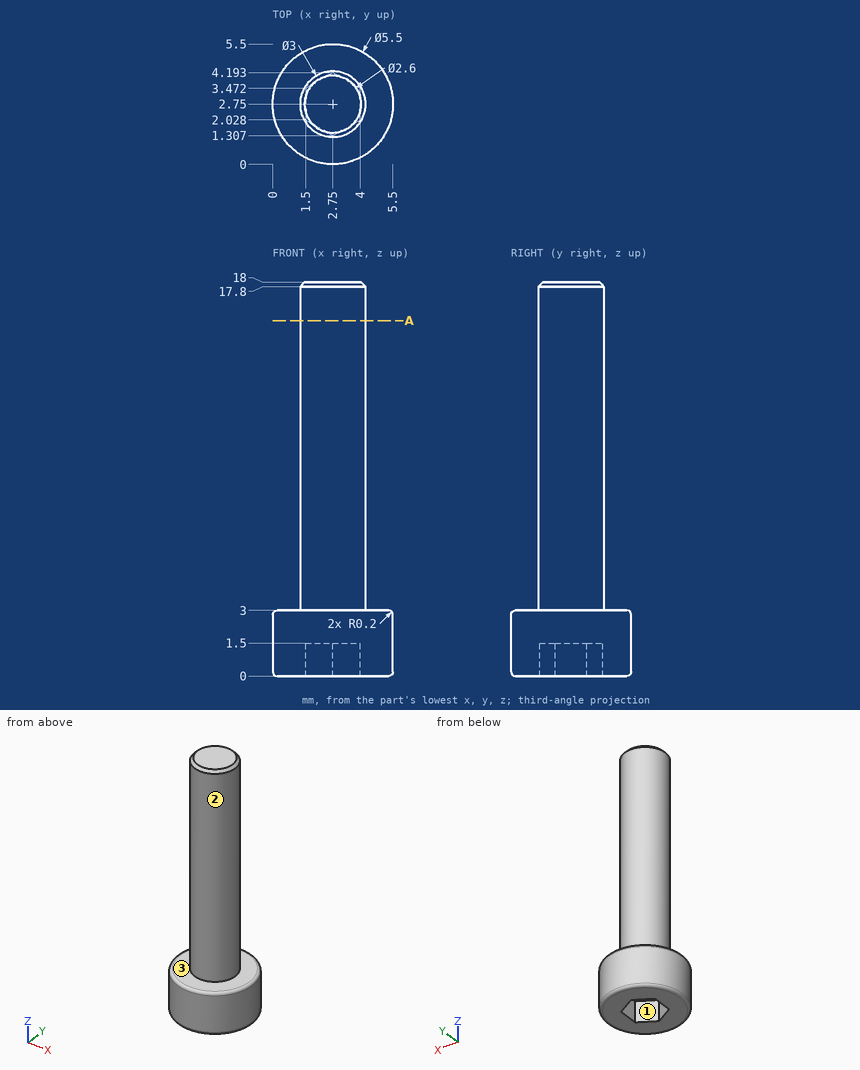
Here's the drawing with two shaded views (mm, measured from the low corner). I have some questions. Give positions to 0.01 mm unless a question says otherwise; leave off trailing zeros. Order: outer loops, then holes, each group sorted by start corner. A loop starts at its lowest first (then second) coordinate and runs counter-clockwise, first axis right, second up.
Q1. If I drill on line 1 along Z through (x, y) = (0.85, 4.4); line 2 along Z through (x, y) = (1.9, 2); line 3 along Y through (x, z) = (3.5, 2.5) (1 decimal), over which ranges is the centre line in solid material (lowest first)?
Q2. We'd pull the mould along X, two halves only. Please class the marked faces 1, 2 and 3: +X half, -X half, draft (parallel to the pull), parting line (faces both ways), or undercut.
Q3. I'm going to push flat-ended pins straight in: P1, Ø1.3, axis at x = 2.5, y = 2.5, coming from the -Z side; P2, Ø1, axis at x = 1.5, z = 7.5, coming from the -Y side; P3, Ø1.5, axis at y = 3, z = 12, coming from the +X side. Where does each tip first touch, or does it pass through?
Q4. Suppose I cut it at A-A, the plane z = 16.25. Write out the boundary of the cut face in (x, y).
Solution:
1. line 1: z = 0 to 3
1. line 2: z = 1.5 to 18
1. line 3: y = 0.1 to 5.4
2. face 1: undercut
2. face 2: parting line
2. face 3: draft
3. P1: stops at z = 1.5
3. P2: stops at y = 1.45
3. P3: stops at x = 4.25
4. outline: circle Ø3 at (2.75, 2.75)
